Autodesk Inventor part; units mm, degrees
ref_plane "YZ Plane" through (0, 0, 0) normal (1, 0, 0) x (0, 1, 0)
ref_plane "XZ Plane" through (0, 0, 0) normal (0, 1, 0) x (-1, 0, 0)
ref_plane "XY Plane" through (0, 0, 0) normal (0, 0, 1) x (1, 0, 0)
sketch "Sketch1" plane through (0, 0, 0) normal (0, 0, 1) x (1, 0, 0)
  line L0 (0, 0) -> (25.4, 0)
  line L1 (25.4, 0) -> (25.4, 25.4)
  line L2 (25.4, 25.4) -> (0, 25.4)
  line L3 (0, 25.4) -> (0, 0)
  dimension "d0" = 25.4
  dimension "d1" = 25.4
extrude "Extrusion1" add sketch "Sketch1" along normal blind 127
shell "Shell1" thickness 3.175 removed faces 2 at (8.4667, 16.9333, 0) at (8.4667, 16.9333, 127)
sketch "Sketch2" plane through (0, 25.4, 0) normal (0, 1, 0) x (1, 0, 0)
  circle A0 centre (12.7, -12.7) radius 1.9685
  line L0 (0, 0) -> (0, -127)
  line L1 (25.4, 0) -> (0, 0)
  circle A1 centre (12.7, -38.1) radius 1.9685
  circle A2 centre (12.7, -63.5) radius 1.9685
  circle A3 centre (12.7, -88.9) radius 1.9685
  circle A4 centre (12.7, -114.3) radius 1.9685
  dimension "d5" = 3.937
  dimension "d6" = 12.7
  dimension "d7" = 12.7
  dimension "d10" = 25.4
extrude "Extrusion2" cut sketch "Sketch2" against normal blind 127
sketch "Sketch3" plane through (25.4, 0, 0) normal (1, 0, 0) x (0, 0, -1)
  circle A0 centre (-12.7, 12.7) radius 1.9685
  line L0 (0, 25.4) -> (-127, 25.4)
  line L1 (0, 0) -> (0, 25.4)
  circle A1 centre (-38.1, 12.7) radius 1.9685
  circle A2 centre (-63.5, 12.7) radius 1.9685
  circle A3 centre (-88.9, 12.7) radius 1.9685
  circle A4 centre (-114.3, 12.7) radius 1.9685
  dimension "d17" = 3.937
  dimension "d18" = 12.7
  dimension "d19" = 12.7
  dimension "d22" = 25.4
extrude "Extrusion3" cut sketch "Sketch3" against normal blind 127
properties part number "Kermit Frame 12"
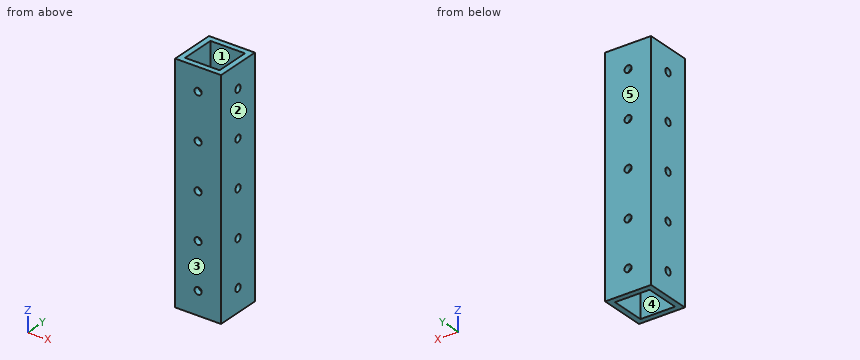
Here's how the part is built. I have some questions about the finished solid (model axes, mm). Face numbers are marked on the shaded views. A direction names the side the tool comes from. Coordinates: 2 decimals unless noted, no trailing zeros. Write each loop counter-clockwise with the first axis right and the second up, starting at its lowest first coordinate (ties: lowest second). Pieces come first, ordered by that corner, then holes. Notation, with made-up numbers: (20, -23.5) - (68, -23.5) arc R29 ccw to (68, -1.5) - close; hole circle Ø11 at (7.5, -2.75). An arc over 180 degrees is marked (long way). Use one line per item in the form item = value.
1) I'm going to push a flat-ended pin straight in: P1, Ø2.5, axis at x = 12.7, z = 88.9, coming from the +Y side. Where does the tip first touch, or does it pass through?
Solved:
P1 = through
2) Suppose I cut it at C-C, the plane z = 101. Write out the boundary of the cut face in (x, y) (3 decimals).
Solved:
outline = (0, 0) - (25.4, 0) - (25.4, 25.4) - (0, 25.4) - close; hole (3.175, 3.175) - (22.225, 3.175) - (22.225, 22.225) - (3.175, 22.225) - close
3) Suppose I cut it at A-A, the plane x = 18.75. Write out the boundary of the cut face in (y, z) (3 decimals).
Solved:
outline = (0, 0) - (3.175, 0) - (3.175, 127) - (0, 127) - close; (22.225, 0) - (25.4, 0) - (25.4, 127) - (22.225, 127) - close
4) Thinking about a two-plate mould opening in X: for the marked faces 1, 2 and 3, which applies, released by +X, released by -X, zero draft, split by the parting line, or undercut?
Solved:
face_1 = undercut
face_2 = released by +X
face_3 = zero draft
5) I need wall thicknesses on line 1 (Z direction, x = 12.7, y = 23.05); line 2 (X direction, y = 19.75, z = 75) (3 decimals); line 3 (X direction, y = 2.1, z = 12.7). Which ranges of each line are inside material? Lowest first, please.
Solved:
line_1 = 0 to 10.73, 14.67 to 36.13, 40.07 to 61.53, 65.47 to 86.93, 90.87 to 112.33, 116.27 to 127
line_2 = 0 to 3.175, 22.225 to 25.4
line_3 = 0 to 10.73, 14.67 to 25.4
6) On a 3-axis mill with a long thin cutter (end or side, diameter ignored), from which of +Z, -Z, +X, -X, +Y, -Y can I reach the whole of each face in a straight line? I mean the marked faces 4 and 5. Say none if no direction works.
Solved:
face_4 = +Z, -Z
face_5 = +Z, -Z, +X, -X, +Y
7) Suppose I cut it at D-D, the plane z = 12.7. Write out the boundary of the cut face in (x, y) (1 decimal), plus the area to 3 significant figures.
Solved:
outline = (0, 0) - (10.7, 0) - (10.7, 3.2) - (3.2, 3.2) - (3.2, 10.7) - (0, 10.7) - close; (0, 14.7) - (3.2, 14.7) - (3.2, 22.2) - (10.7, 22.2) - (10.7, 25.4) - (0, 25.4) - close; (14.7, 0) - (25.4, 0) - (25.4, 10.7) - (22.2, 10.7) - (22.2, 3.2) - (14.7, 3.2) - close; (14.7, 22.2) - (22.2, 22.2) - (22.2, 14.7) - (25.4, 14.7) - (25.4, 25.4) - (14.7, 25.4) - close
area = 232 mm2
